```python
from build123d import *

# Parameters (mm, degrees)
BOSS_EXTRUDE1_DEPTH = 6
SKETCH4_R           = 1.5
CUT_EXTRUDE1_DEPTH  = 3


with BuildPart() as part:
    # Sketch1 → Boss-Extrude1 (new body)
    with BuildSketch(Plane.XY):
        Polygon((0, 0), (-20, 0), (-20, -20), (-17, -20), (-17, -3), (0, -3), align=None)
    extrude(amount=BOSS_EXTRUDE1_DEPTH)

    # Sketch4 → Cut-Extrude1 (cut)
    with BuildSketch(Plane.ZY.offset(20)):
        with Locations((3, -7)):
            Circle(SKETCH4_R)
        with Locations((3, -17)):
            Circle(SKETCH4_R)
    extrude(amount=-CUT_EXTRUDE1_DEPTH, mode=Mode.SUBTRACT)


solid = part.part
```
Geometry: final body of the model. Coordinates: model frame, mm. A direction names the side the tool comes from. Round coordinates to 2 decimals unless told otherwise and drop trailing zeros. Write each loop counter-clockwise with the first axis right and the second up, starting at its lowest first coordinate (ties: lowest second). Pieces come first, ordered by that corner, then holes.
Item 1: Mould query, pull axis Y, two halves, no side actions, for faces 3 (the face through (-18.521, -15.735, 3.806)), 4 (the face through (-14.5, -2.5, 0)), 5 (the face through (-10, 0, 3)). Classes: +Y half, -Y half, draft (parallel to the pull), parting line (faces both ways), or undercut.
Item 2: Section query B-B (z = 3). Return loops of the section in (x, y).
Item 3: Section query C-C (x = -17.25). Return loops of the section in (y, z), plus the area to 3 significant figures.
Item 4: Set-up query: faces 1 (the face through (-19, -20, 3)), 2 (the face through (-17, -12, 3)). Return all of +Z, -Z, +X, -X, +Y, -Y with unobstructed straight access to the full face (end or side cutting, diameter ignored); none if empty.
Item 5: Section query D-D (z = 0.8). Return loops of the section in (x, y).
Item 6: Section query A-A (y = -17). Return loops of the section in (x, z), plus the area to 3 significant figures.
Item 7: Pin query (flat end, axial travel): P1, Ø1.5, axis at y = -6.5, z = 2.5, coming from the -X side; P2, Ø3, axis at x = -12, z = 3, coming from the -Y side. Return the tip coordinate at first contact, or that it passes through.
Item 8: Material intervals for L1, parallel to Y at x = -17.8, z = 3; L2, parallel to X at y = -14.75, z = 2.2; L3, parallel to Y at x = -0.75, z = 2.4, sorted ascending.
Completed:
1. face 3: undercut
1. face 4: draft
1. face 5: +Y half
2. outline: (-20, -20) - (-17, -20) - (-17, -18.5) - (-20, -18.5) - close; (-20, -15.5) - (-17, -15.5) - (-17, -8.5) - (-20, -8.5) - close; (-20, -5.5) - (-17, -5.5) - (-17, -3) - (0, -3) - (0, 0) - (-20, 0) - close
3. outline: (-20, 0) - (0, 0) - (0, 6) - (-20, 6) - close; hole circle Ø3 at (-17, 3); hole circle Ø3 at (-7, 3)
3. area: 106 mm2
4. face 1: +Z, -Z, +X, -X, -Y
4. face 2: +Z, -Z, +X, -Y
5. outline: (-20, -20) - (-17, -20) - (-17, -3) - (0, -3) - (0, 0) - (-20, 0) - close
6. outline: (-20, 0) - (-17, 0) - (-17, 1.5) - (-20, 1.5) - close; (-20, 4.5) - (-17, 4.5) - (-17, 6) - (-20, 6) - close
6. area: 9.00 mm2
7. P1: passes through
7. P2: stops at y = -3
8. L1: y = -20 to -18.5, -15.5 to -8.5, -5.5 to 0
8. L2: x = -20 to -17
8. L3: y = -3 to 0
